Build history of the part. All positions in model axes, mm. A direction names the side the tool comes from. Coordinates: 2 decimals unless noted, no trailing zeros. Order: outer loops, then holes, each group sorted by start corner. A loop starts at its lowest first (then second) coordinate and runs counter-clockwise, first axis right, second up. Notation, with made-up numbers: (1, 73.25) -> (22, 73.25) arc R30 cw to (22, 102.25) -> close; hole circle Ø11 at (78.25, 25.5). An arc over 180 degrees is marked (long way). Write each question's results on one line, items separated by ' | '.
from build123d import *

# Parameters (mm, degrees)
SKETCH1_R           = 4.05
SKETCH1_W           = 5.3
SKETCH1_H           = 3.8
BOSS_EXTRUDE1_DEPTH = 6
BOSS_EXTRUDE2_DEPTH = 1.5
SKETCH3_R           = 0.9
SKETCH3_W           = 5.3
SKETCH3_H           = 3.8
CUT_EXTRUDE1_DEPTH  = 1.5


with BuildPart() as part:
    # Sketch1 → Boss-Extrude1 (new body)
    with BuildSketch(Plane(origin=(0, 0, 0), x_dir=(1, 0, 0), z_dir=(0, 1, 0))):
        with Locations(Location((0, 0, 0), (0, 0, 270))):
            Circle(SKETCH1_R)
        Rectangle(SKETCH1_W, SKETCH1_H, mode=Mode.SUBTRACT)
    extrude(amount=BOSS_EXTRUDE1_DEPTH)

    # Sketch2 → Boss-Extrude2 (add)
    with BuildSketch(Plane(origin=(0, 0, 0), x_dir=(1, 0, 0), z_dir=(0, 1, 0))):
        with BuildLine():
            Line((-18, 1.8), (0, 4.05))
            Line((0, 4.05), (18, 1.8))
            ThreePointArc((18, 1.8), (19.8, 0), (18, -1.8))
            Line((18, -1.8), (0, -4.05))
            Line((0, -4.05), (-18, -1.8))
            ThreePointArc((-18, -1.8), (-19.8, 0), (-18, 1.8))
        make_face()
    extrude(amount=BOSS_EXTRUDE2_DEPTH)

    # Sketch3 → Cut-Extrude1 (cut)
    with BuildSketch(Plane(origin=(0, 0, 0), x_dir=(1, 0, 0), z_dir=(0, 1, 0))):
        with Locations(Location((-17.1, 0, 0), (0, 0, 270))):
            Circle(SKETCH3_R)
        with Locations(Location((17.1, 0, 0), (0, 0, 270))):
            Circle(SKETCH3_R)
        Rectangle(SKETCH3_W, SKETCH3_H)
    extrude(amount=CUT_EXTRUDE1_DEPTH, mode=Mode.SUBTRACT)


solid = part.part
Item 1: Pin check, flat tips, straight feed: pin 1 (1.9 mm diameter, centred on y = 3.5, z = 1, fed in from -X); pin 2 (1.6 mm diameter, centred on x = -17.1, z = 0, fed in from -Y); pin 3 (1 mm diameter, centred on y = 5, z = -3, fed in from +X); pin 4 (1.1 mm diameter, centred on y = 3.5, z = 0.5, fed in from +X). Stop position of each tip, or through.
Answer:
pin 1: stops at x = -4.05 | pin 2: passes through | pin 3: stops at x = 3.19 | pin 4: stops at x = 4.05
Item 2: Slice it at B-B, the plane z = 0. List the corners of the cut face in (x, y).
Answer:
outline: (-19.8, 0) -> (-18, 0) -> (-18, 1.5) -> (-19.8, 1.5) -> close; (-16.2, 0) -> (-2.65, 0) -> (-2.65, 6) -> (-4.05, 6) -> (-4.05, 1.5) -> (-16.2, 1.5) -> close; (2.65, 0) -> (16.2, 0) -> (16.2, 1.5) -> (4.05, 1.5) -> (4.05, 6) -> (2.65, 6) -> close; (18, 0) -> (19.8, 0) -> (19.8, 1.5) -> (18, 1.5) -> close
Item 3: Slice it at A-A, the plane y = 0.85. List the corners of the cut face in (x, z), and give its area (3 significant figures).
Answer:
outline: (-18, -1.8) -> (-1, -3.93) arc R4.05 ccw to (1, -3.93) -> (18, -1.8) arc R1.8 ccw to (18, 1.8) -> (1, 3.93) arc R4.05 ccw to (-1, 3.93) -> (-18, 1.8) arc R1.8 ccw to start; hole circle Ø1.8 at (-17.1, 0); hole (-2.65, -1.9) -> (2.65, -1.9) -> (2.65, 1.9) -> (-2.65, 1.9) -> close; hole circle Ø1.8 at (17.1, 0) | area: 196 mm^2
Item 4: Slice it at D-D, the plane y = 5.15. List the corners of the cut face in (x, z), and give its area (3 significant figures).
Answer:
outline: circle Ø8.1 at (0, 0); hole (-2.65, -1.9) -> (2.65, -1.9) -> (2.65, 1.9) -> (-2.65, 1.9) -> close | area: 31.4 mm^2
Item 5: Tool access for faces 1 (the cylindrical face through (0.178, 3.625, -4.046)), 2 (the flat face through (9.617, 0.74, 2.848)), 3 (the flat face through (-2.65, 3, 0)): list every direction of +Z, -Z, +X, -X, +Y, -Y with a clear straight run to the whole face (end or side of a thin tool).
Answer:
face 1: +Y | face 2: +Z, +X, +Y, -Y | face 3: +Y, -Y
Item 6: Slice it at C-C, the plane x = 17.1. List the corners of the cut face in (y, z), and give its area (3 significant figures).
Answer:
outline: (0, -1.91) -> (1.5, -1.91) -> (1.5, -0.9) -> (0, -0.9) -> close; (0, 0.9) -> (1.5, 0.9) -> (1.5, 1.91) -> (0, 1.91) -> close | area: 3.04 mm^2
Item 7: Drill centre lines: line 1 (X direction, y = 1.15, z = 0); line 2 (X direction, y = 2.7, z = 1); line 3 (Z direction, x = 1, y = 4.4). Where is each one in solid material? Low to high. Write a range as from..to.
Answer:
line 1: x = -19.8..-18, -16.2..-2.65, 2.65..16.2, 18..19.8 | line 2: x = -3.92..-2.65, 2.65..3.92 | line 3: z = -3.92..-1.9, 1.9..3.92
Item 8: Pull direction Z, two halves, no side cores. Call faces 4 (the flat face through (-9.379, 0.74, 2.878)), 5 (the cylindrical face through (-16.21, 0.74, -0.12)), 6 (the flat face through (0, 0, 3)), 7 (the flat face through (0, 3, -1.9)): released by +Z, released by -Z, zero draft, split by the parting line, or undercut.
Answer:
face 4: released by +Z | face 5: undercut | face 6: zero draft | face 7: undercut
